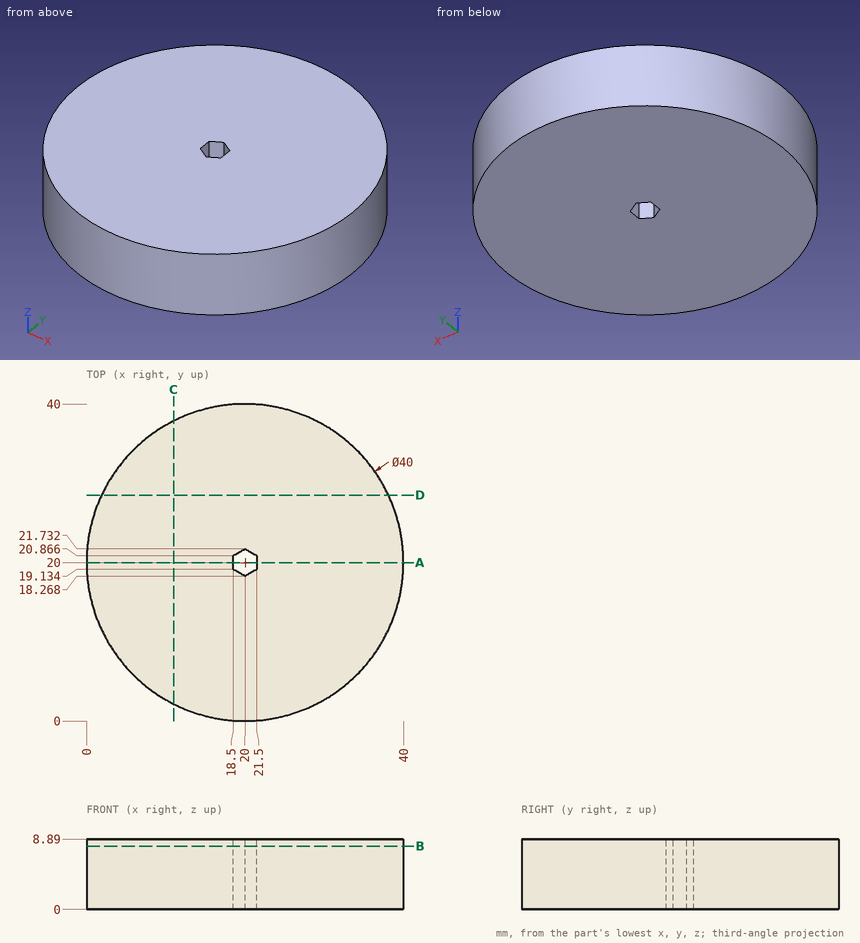
Source: three-view drawing plus pictorial views. Frame: mm from the lowest corner of the part. Round coordinates to 2 decimals unless told otherwise and drop trailing zeros. Order: outer loops, then holes, each group sorted by start corner. A loop starts at its lowest first (then second) coordinate and runs counter-clockwise, first axis right, second up. Notation, with made-up numbers: (-6, 40.5) - (8, 40.5) arc R33 cw to (8, 69.5) - close; hole circle Ø4 at (25.25, 26). An arc over 180 degrees is marked (long way). Write each question's results on one line, items separated by ' | '.
Item 1: Material intervals for line 1 along X through (y, z) = (21, 1.5) (1 decimal); line 2 along X through (y, z) = (22, 7.5); line 3 along Y through (x, z) = (13, 4.5) (3 decimals), sorted ascending. Write a range as [from, to].
Completed:
line 1: [0, 18.7], [21.3, 40] | line 2: [0.1, 39.9] | line 3: [1.265, 38.735]
Item 2: Section B-B, the plane z = 8. Return the cut outline in (x, y).
Completed:
outline: circle Ø40 at (20, 20); hole (18.5, 19.13) - (20, 18.27) - (21.5, 19.13) - (21.5, 20.87) - (20, 21.73) - (18.5, 20.87) - close
Item 3: Section C-C, the plane x = 11. Return the cut outline in (y, z).
Completed:
outline: (2.14, 0) - (37.86, 0) - (37.86, 8.89) - (2.14, 8.89) - close
Item 4: First-contact query: pin 1 Ø1 at (x, z) = (6, 7) entering from -Y; pin 2 Ø4 at (x, z) = (5.5, 3) entering from +Y; pin 3 Ø3 at (y, z) = (14.5, 3) entering from +X; pin 4 Ø1 at (x, y) = (32.5, 19.5) entering from -Z. Flat tips, straight axial feed; report the tip coordinate or a pass-through.
Completed:
pin 1: y = 5.24 | pin 2: y = 35.61 | pin 3: x = 39.6 | pin 4: z = 0
Item 5: Section A-A, the plane y = 20. Return the cut outline in (x, z).
Completed:
outline: (0, 0) - (18.5, 0) - (18.5, 8.89) - (0, 8.89) - close; (21.5, 0) - (40, 0) - (40, 8.89) - (21.5, 8.89) - close
Item 6: Section D-D, the plane y = 28.5. Return the cut outline in (x, z), and give its area (3 significant figures).
Completed:
outline: (1.9, 0) - (38.1, 0) - (38.1, 8.89) - (1.9, 8.89) - close | area: 322 mm^2
